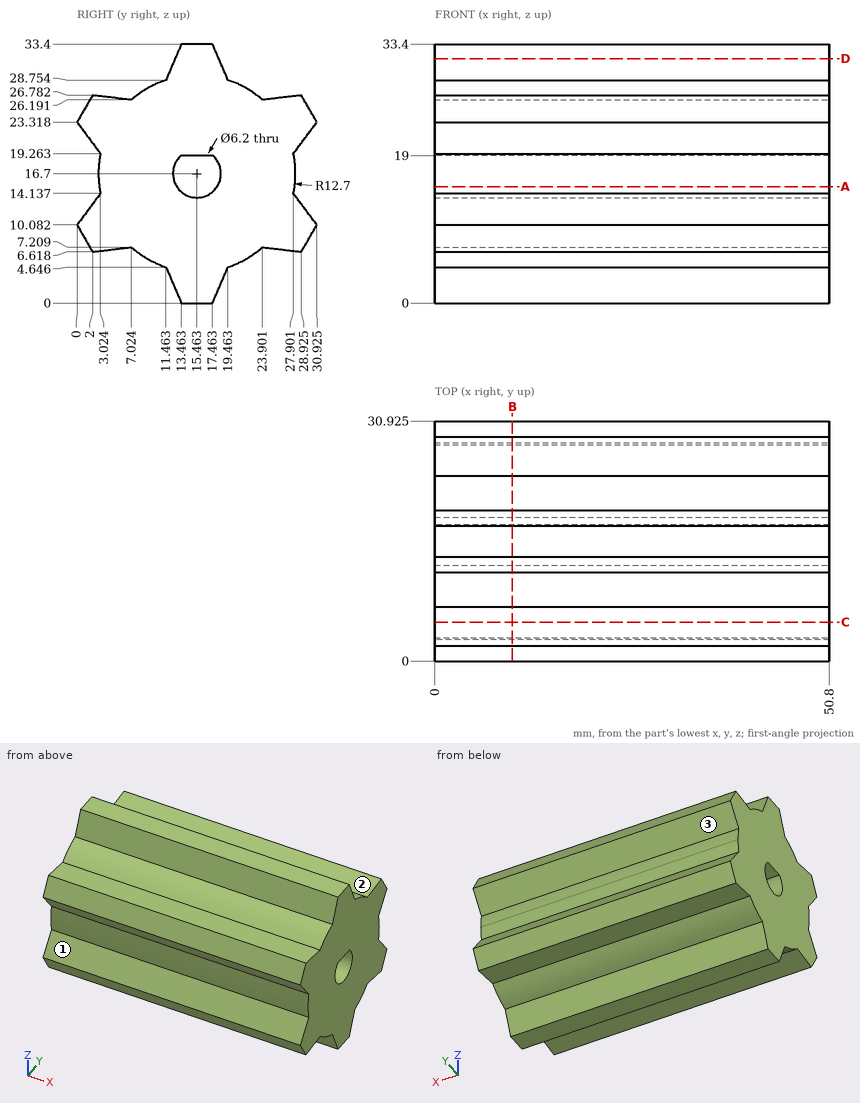
Input: dimensioned drawing with shaded views. Units: mm. Origin: part minimum x, y, z. A direction names the side the tool comes from. Coordinates: 2 decimals unless noted, no trailing zeros. Loops run counter-clockwise (first coordinate to the right, second up) from the corner with the lowest first, then second, coordinate; pieces in that order, holes last. Notation, with made-up numbers: M 86,10 L 128,10 A27 cw 128,37 Z; hole C 88,49.5 d10. An arc over 180 degrees is marked long. Use a Markdown table: item, result. Add a question column.
Q1. Section query B-B, the plane x = 10. Return loops of the section in (y, z) (1 decimal), and give its area (3 significant figures).
Q2. Section query A-A, the plane z = 15. Return loops of the section in (x, y) (1 decimal), and give its area (3 significant figures).
Q3. Section query C-C, the plane y = 5. Return loops of the section in (x, z).
Q4. Material intervals for L1, parallel to Y at x = 18, z = 16.7; L2, parallel to Y at x = 25, z = 16; L3, parallel to Z at x = 10, y = 14 (1 decimal), sorted ascending.
Q5. Section query D-D, the plane z = 31.5. Return loops of the section in (x, y) (1 decimal), and give its area (3 significant figures).
Q6. First-contact query: pin 1 (8 mm diameter, centred on x = 23, y = 7.5, fed in from +Z); pin 2 (2 mm diameter, centred on x = 28, z = 5, fed in from +Y) (1 decimal); pin 3 (1 mm diameter, centred on x = 43, z = 12, fed in from -Y). Flat tips, straight axial feed; report the tip coordinate or a pass-through.
Q7. Access query for the marked faces 1, 2 and 3. Directions: +Z, -Z, +X, -X, +Y, -Y. A direction counts if a zero-diameter tool reaches every point of the face in a straight line with its end or side. Return the directions, or none.
Result:
| question | item | result |
|---|---|---|
| 1 | outline | M 0,10.1 L 2,6.6 L 7,7.2 A12.7 ccw 11.5,4.6 L 13.5,0 L 17.5,0 L 19.5,4.6 A12.7 ccw 23.9,7.2 L 28.9,6.6 L 30.9,10.1 L 27.9,14.1 A12.7 ccw 28.2,16.7 A12.7 ccw 27.9,19.3 L 30.9,23.3 L 28.9,26.8 L 23.9,26.2 A12.7 ccw 19.5,28.8 L 17.5,33.4 L 13.5,33.4 L 11.5,28.8 A12.7 ccw 7,26.2 L 2,26.8 L 0,23.3 L 3,19.3 A12.7 ccw 3,14.1 Z; hole M 13.4,19 A3.1 ccw long 17.5,19 Z |
| 1 | area | 625 mm2 |
| 2 | outline | M 0,2.9 L 50.8,2.9 L 50.8,12.9 L 0,12.9 Z; M 0,18.1 L 50.8,18.1 L 50.8,28 L 0,28 Z |
| 2 | area | 1,020 mm2 |
| 3 | outline | M 0,6.97 L 50.8,6.97 L 50.8,26.43 L 0,26.43 Z |
| 4 | L1 | y = 2.76 to 12.36, 18.56 to 28.16 |
| 4 | L2 | y = 2.78 to 12.44, 18.48 to 28.14 |
| 4 | L3 | z = 0 to 14, 19 to 33.4 |
| 5 | outline | M 0,12.6 L 50.8,12.6 L 50.8,18.3 L 0,18.3 Z |
| 5 | area | 286 mm2 |
| 6 | pin 1 | stops at z = 28.84 |
| 6 | pin 2 | stops at y = 22.3 |
| 6 | pin 3 | stops at y = 1.06 |
| 7 | face 1 | +X, -X, -Y |
| 7 | face 2 | +Z, +X, -X |
| 7 | face 3 | +X, -X, +Y |
